Can you work these out from the model? Positions are in its coordinate system, mm. Round coordinates to 2 decimals unless told otherwise and drop trailing zeros. Write each loop counter-clockwise with the first axis right and the second up, starting at its lowest first coordinate (ties: lowest second). Pieces come first, ordered by that corner, then holes.
Q1. If we section it at D-D (x = 105.41): Please give me the cut outline in (y, z) (3 decimals).
Q2. We'd pull the mould along X, two halves only. Please class faces 1 (the cylindrical face through (49.38, 98, 6.44)), 2 (the flat face through (-2, -17, 12.7)), 3 (the cylindrical face through (102.15, -57.01, 6.44)), 4 (the flat face through (-130.175, -52, 6)): +X half, -X half, draft (parallel to the pull), parting line (faces both ways), or undercut.
Q3. If we section it at A-A (y = -57.15): Please give me the cut outline in (x, z) (3 decimals).
Q4. If we section it at B-B (x = 0): Please give me the cut outline in (y, z) (3 decimals), plus the area to 3 significant figures.
Q5. If we section it at C-C (z = 4.25): Give the number of separate pieces and of enclosed holes in the cut face, plus the area to 3 significant figures.
Q6. I'm going to push a flat-ended pin straight in: pin 1 Ø2.5 at (x, y) = (60.325, -120.65) entering from +Z. Where does the tip first touch, or does it pass through?
Q7. Please list where these lines run through material, in increasing order: line 1 along Y through (x, z) = (-50.8, 7.5) (3 decimals); line 2 along Y through (x, z) = (105.41, 8.75) (3 decimals); line 3 along X through (y, z) = (96.5, 10).
from build123d import *

# Parameters (mm, degrees)
BOSS_EXTRUDE1_DEPTH         = 12.7
SKETCH2_R                   = 19.05
CUT_EXTRUDE1_DEPTH          = 214.127417875
F_16_0_177_DIAMETER_HOLE1_D = 4.4958
F_0_257_DIAMETER_HOLE1_D    = 6.5278


with BuildPart() as part:
    # Sketch1 → Boss-Extrude1 (new body)
    with BuildSketch(Plane.XY):
        Polygon((-130.175, -168.275), (130.175, -168.275), (130.175, 60.325), (60.325, 130.175), (-60.325, 130.175), (-130.175, 60.325), align=None)
    extrude(amount=BOSS_EXTRUDE1_DEPTH)

    # Sketch2 → Cut-Extrude1 (cut, through all)
    with BuildSketch(Plane.XY):
        with Locations((0, -57.15)):
            Circle(SKETCH2_R)
    extrude(amount=CUT_EXTRUDE1_DEPTH, mode=Mode.SUBTRACT)

    # #16 (0.177) Diameter Hole1 (through all)
    with Locations(Plane.XY.offset(12.7)):
        with Locations((-50.8, 115.9002), (50.8, 115.9002), (119.0752, 11.1252), (119.0752, -63.5), (60.325, -120.65), (-19.05, -134.9375), (-92.075, -98.425), (-119.0752, 11.1252)):
            Hole(F_16_0_177_DIAMETER_HOLE1_D / 2)

    # F (0.257) Diameter Hole1 (through all)
    with Locations(Plane(origin=(0, 0, 0), x_dir=(-1, 0, 0), z_dir=(0, 0, -1))):
        with Locations((-105.41, -57.15), (-93.98, 60.325), (-47.625, 95.25)):
            Hole(F_0_257_DIAMETER_HOLE1_D / 2)


solid = part.part
A:
1. outline: (-168.275, 0) - (-60.414, 0) - (-60.414, 12.7) - (-168.275, 12.7) - close; (-53.886, 0) - (85.09, 0) - (85.09, 12.7) - (-53.886, 12.7) - close
2. face 1: undercut
2. face 2: draft
2. face 3: undercut
2. face 4: -X half
3. outline: (-130.175, 0) - (-19.05, 0) - (-19.05, 12.7) - (-130.175, 12.7) - close; (19.05, 0) - (102.146, 0) - (102.146, 12.7) - (19.05, 12.7) - close; (108.674, 0) - (130.175, 0) - (130.175, 12.7) - (108.674, 12.7) - close
4. outline: (-168.275, 0) - (-76.2, 0) - (-76.2, 12.7) - (-168.275, 12.7) - close; (-38.1, 0) - (130.175, 0) - (130.175, 12.7) - (-38.1, 12.7) - close
4. area: 3,310 mm2
5. separate pieces: 1
5. enclosed holes: 12
5. area: 71,500 mm2
6. pin 1: passes through
7. line 1: y = -168.275 to 113.652, 118.148 to 130.175
7. line 2: y = -168.275 to -60.414, -53.886 to 85.09
7. line 3: x = -94 to 44.61, 50.64 to 94
